```python
from build123d import *

# Parameters (mm, degrees)
ESQUISSE1_R                         = 150
BASE_CIRCULAIRE_DEPTH               = 5
ESQUISSE2_W                         = 20
ESQUISSE2_H                         = 80
EMPLACEMENT_ROUES_DEPTH             = 6
ESQUISSE3_R                         = 1.5
ESQUISSE3_R_2                       = 1.575487657
TROUS_FIXATION_MORS_DEPTH           = 6
ESQUISSE4_R                         = 1.5
TROUS_FIXATION_PAROIS_DEPTH         = 6
ESQUISSE5_R                         = 1
TROUS_FIXATION_ROUES_FOLLES_DEPTH   = 6
ESQUISSE6_R                         = 1.59
TROUS_FIXATION_CARTE_OPEN_UPS_DEPTH = 6


with BuildPart() as part:
    # Esquisse1 → base_circulaire (new body)
    with BuildSketch(Plane.XY):
        Circle(ESQUISSE1_R)
    extrude(amount=BASE_CIRCULAIRE_DEPTH)

    # Esquisse2 → emplacement_roues (cut, through all)
    with BuildSketch(Plane.XY.offset(5)):
        with Locations((-110, 0)):
            Rectangle(ESQUISSE2_W, ESQUISSE2_H)
        with Locations((110, 0)):
            Rectangle(ESQUISSE2_W, ESQUISSE2_H)
    extrude(amount=-EMPLACEMENT_ROUES_DEPTH, mode=Mode.SUBTRACT)

    # Esquisse3 → trous_fixation_mors (cut, through all)
    with BuildSketch(Plane.XY.offset(5)):
        with Locations((-85, 35)):
            Circle(ESQUISSE3_R)
        with Locations((-85, -35)):
            Circle(ESQUISSE3_R)
        with Locations((85, 35)):
            Circle(ESQUISSE3_R)
        with Locations((85, -35)):
            Circle(ESQUISSE3_R)
        with Locations((65, -35)):
            Circle(ESQUISSE3_R_2)
        with Locations((65, 35)):
            Circle(ESQUISSE3_R)
        with Locations((-65, -35)):
            Circle(ESQUISSE3_R)
        with Locations((-65, 35)):
            Circle(ESQUISSE3_R)
    extrude(amount=-TROUS_FIXATION_MORS_DEPTH, mode=Mode.SUBTRACT)

    # Esquisse4 → trous fixation parois (cut, through all)
    with BuildSketch(Plane.XY.offset(5)):
        with Locations((-102.530483272, 95.45941546)):
            Circle(ESQUISSE4_R)
        with Locations((-95.45941546, 102.530483272)):
            Circle(ESQUISSE4_R)
        with Locations((95.45941546, 102.530483272)):
            Circle(ESQUISSE4_R)
        with Locations((102.530483272, 95.45941546)):
            Circle(ESQUISSE4_R)
        with Locations((102.530483272, -95.45941546)):
            Circle(ESQUISSE4_R)
        with Locations((95.45941546, -102.530483272)):
            Circle(ESQUISSE4_R)
        with Locations((-95.45941546, -102.530483272)):
            Circle(ESQUISSE4_R)
        with Locations((-102.530483272, -95.45941546)):
            Circle(ESQUISSE4_R)
    extrude(amount=-TROUS_FIXATION_PAROIS_DEPTH, mode=Mode.SUBTRACT)

    # Esquisse5 → trous fixation roues folles (cut, through all)
    with BuildSketch(Plane.XY.offset(5)):
        with Locations((8.947, 126.053)):
            Circle(ESQUISSE5_R)
        with Locations((8.947, 131.947)):
            Circle(ESQUISSE5_R)
        with Locations((-8.947, 126.053)):
            Circle(ESQUISSE5_R)
        with Locations((-8.947, 131.947)):
            Circle(ESQUISSE5_R)
        with Locations((8.947, -131.947)):
            Circle(ESQUISSE5_R)
        with Locations((-8.947, -131.947)):
            Circle(ESQUISSE5_R)
        with Locations((8.947, -126.053)):
            Circle(ESQUISSE5_R)
        with Locations((-8.947, -126.053)):
            Circle(ESQUISSE5_R)
    extrude(amount=-TROUS_FIXATION_ROUES_FOLLES_DEPTH, mode=Mode.SUBTRACT)

    # Esquisse6 → trous fixation carte open UPS (cut, through all)
    with BuildSketch(Plane.XY.offset(5)):
        with Locations((46.005, 65)):
            Circle(ESQUISSE6_R)
        with Locations((46.005, 112.01)):
            Circle(ESQUISSE6_R)
        with Locations((-46.005, 65)):
            Circle(ESQUISSE6_R)
        with Locations((-46.005, 112.01)):
            Circle(ESQUISSE6_R)
    extrude(amount=-TROUS_FIXATION_CARTE_OPEN_UPS_DEPTH, mode=Mode.SUBTRACT)


solid = part.part
```
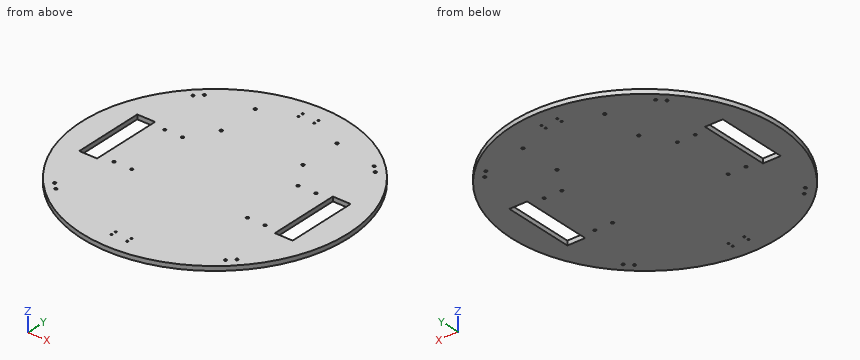
Model file for the job. Use its own axes, mm. Coordinates: 2 decimals unless noted, no trailing zeros. Write each loop counter-clockwise with the first axis right and the second up, starting at its lowest first coordinate (ties: lowest second). Pieces come first, ordered by that corner, then holes. Notation, with made-up numbers: (-32.5, 78.5) - (4.5, 78.5) arc R17 cw to (4.5, 110.5) - close; hole circle Ø2 at (57, -29.75). An arc over 180 degrees is marked (long way). One line per item, written item: value. Start each with the question number.
1. Slice it at B-B (x = 27). Write the cut outline in (y, z), plus the area to 3 significant figures.
2. Slice it at A-A (y = 0). Write the cut outline in (x, z).
3. Slice it at D-D (x = -35.5). Write the cut outline in (y, z).
4. Slice it at C-C (z = 4.2). Count the separate pieces of the cut face and the enclosed holes in it, plus the area to 3 significant figures.
5. Probe line 1 (X direction, y = 2, z = 0.95); line 2 (Y direction, x = 85, z = 3.7); line 3 (X direction, y = 18.5, z = 2.4). List the from-to ranges inside material, lowest first. Write a range as from..to.
6. Flat gauge pins, fed straight in: pin 1 (3 mm diameter, centred on y = 36, z = 2.5, fed in from +X); pin 2 (2 mm diameter, centred on y = -81, z = 1.5, fed in from -X); pin 3 (1.5 mm diameter, centred on x = 112, z = 3, fed in from -Y); pin 4 (1.8 mm diameter, centred on x = 85, y = 35, fed in from -Z). Where does each tip first touch, or does it go through?
Answers below:
1. outline: (-147.55, 0) - (147.55, 0) - (147.55, 5) - (-147.55, 5) - close
1. area: 1,480 mm^2
2. outline: (-150, 0) - (-120, 0) - (-120, 5) - (-150, 5) - close; (-100, 0) - (100, 0) - (100, 5) - (-100, 5) - close; (120, 0) - (150, 0) - (150, 5) - (120, 5) - close
3. outline: (-145.74, 0) - (145.74, 0) - (145.74, 5) - (-145.74, 5) - close
4. separate pieces: 1
4. enclosed holes: 30
4. area: 67,300 mm^2
5. line 1: x = -149.99..-120, -100..100, 120..149.99
5. line 2: y = -123.59..-36.5, -33.5..33.5, 36.5..123.59
5. line 3: x = -148.85..-120, -100..100, 120..148.85
6. pin 1: stops at x = 145.98
6. pin 2: stops at x = -126.89
6. pin 3: stops at y = -100.62
6. pin 4: passes through
